Design review of the part shown in the three views and the two pictorial views. Dimensions are in mm from the part's minimum x, y and z. Round coordinates to 2 decimals unless told otherwise and drop trailing zeros. Write each loop counter-clockwise with the first axis right and the second up, starting at its lowest first coordinate (ties: lowest second). Pieces come first, ordered by that corner, then holes. Notation, with made-up numbers: (3, 50.5) -> (21, 50.5) arc R16 cw to (21, 68.5) -> close; hole circle Ø3 at (32.5, 42.25). An arc over 180 degrees is marked (long way). Answer as a JSON object with one key per item and string values. Group by question number.
1) To check wall thickness, follow probe 1 along Y at (x, z) = (35, 1.6); probe 2 along Y at (x, z) = (36, 0.3); probe 3 along X at (y, z) = (41.5, 1.65). State the ranges of each line that lie inside material, in increasing order. Write a range as [from, to].
2) We need section D-D, the plane y = 3. Write out the cut boundary in (x, z).
3) We need section A-A, the plane y = 35. Write out the cut boundary in (x, z).
4) Insertion check: pin 1 Ø1 at (x, z) = (48, 1.5) entering from -Y; pin 2 Ø1 at (y, z) = (60.5, 2.5) entering from -X; pin 3 Ø1.5 at (y, z) = (27.5, 0.5) entering from +X. Each pin has a flat end and moves straight along its axis. Give the tip position at first contact, or say it passes through.
5) We need section B-B, the plane z = 1. Write out the cut boundary in (x, y), then the cut area to 3 significant figures.
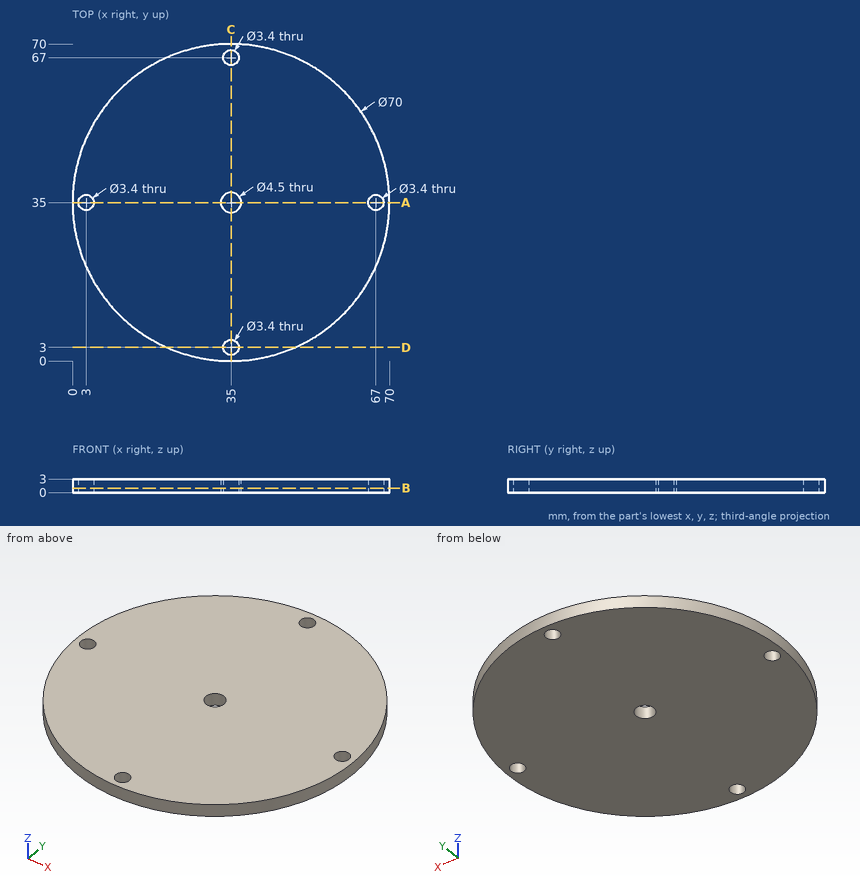
Here are the results:
{
 "1": {"probe 1": "y = [0, 1.3], [4.7, 32.75], [37.25, 65.3], [68.7, 70]", "probe 2": "y = [0.01, 1.63], [4.37, 32.98], [37.02, 65.63], [68.37, 69.99]", "probe 3": "x = [0.61, 69.39]"},
 "2": {"outline": "(20.82, 0) -> (33.3, 0) -> (33.3, 3) -> (20.82, 3) -> close; (36.7, 0) -> (49.18, 0) -> (49.18, 3) -> (36.7, 3) -> close"},
 "3": {"outline": "(0, 0) -> (1.3, 0) -> (1.3, 3) -> (0, 3) -> close; (4.7, 0) -> (32.75, 0) -> (32.75, 3) -> (4.7, 3) -> close; (37.25, 0) -> (65.3, 0) -> (65.3, 3) -> (37.25, 3) -> close; (68.7, 0) -> (70, 0) -> (70, 3) -> (68.7, 3) -> close"},
 "4": {"pin 1": "stops at y = 2.31", "pin 2": "stops at x = 10.51", "pin 3": "stops at x = 69.34"},
 "5": {"outline": "circle Ø70 at (35, 35); hole circle Ø3.4 at (3, 35); hole circle Ø4.5 at (35, 35); hole circle Ø3.4 at (35, 3); hole circle Ø3.4 at (35, 67); hole circle Ø3.4 at (67, 35)", "area": "3,800 mm^2"}
}
